from build123d import *

# Parameters (mm, degrees)
SKETCH1_W           = 200
SKETCH1_H           = 200
BOSS_EXTRUDE1_DEPTH = 340
CAVITY1_START       = -100
CAVITY1_DEPTH       = 200
CAVITY1_START_2     = 91.703376511
CAVITY1_2_DEPTH     = 8.296623489
CAVITY1_3_DEPTH     = 1.703376511


# Read off the part's stored shape, not the designer's step: Cavity1
with BuildPart() as part:
    # Sketch1 → Boss-Extrude1 (new body)
    with BuildSketch(Plane.XY):
        Rectangle(SKETCH1_W, SKETCH1_H)
    extrude(amount=BOSS_EXTRUDE1_DEPTH)

    # Cavity1 outline → Cavity1 (cut)
    with BuildSketch(Plane.YZ.offset(CAVITY1_START)):
        with BuildLine():
            ThreePointArc((100, 19.737266788), (79.748929914, 52.418363447), (64.730256288, 87.81044393))
            Line((64.730256288, 87.81044393), (43.715736742, 87.81044393))
            ThreePointArc((43.715736742, 87.81044393), (31.630726001, 167.81044393), (43.715736742, 247.81044393))
            Line((43.715736742, 247.81044393), (64.730256288, 247.81044393))
            ThreePointArc((64.730256288, 247.81044393), (79.748929914, 283.202524413), (100, 315.883621072))
            Line((100, 315.883621072), (100, 340))
            Line((100, 340), (-100, 340))
            Line((-100, 340), (-100, 0))
            Line((-100, 0), (100, 0))
            Line((100, 0), (100, 19.737266788))
        make_face()
    extrude(amount=CAVITY1_DEPTH, mode=Mode.SUBTRACT)

    # Cavity1 2 outline → Cavity1 2 (cut)
    with BuildSketch(Plane.YZ.offset(CAVITY1_START_2)):
        with BuildLine():
            Line((43.715736742, 87.81044393), (64.730256288, 87.81044393))
            ThreePointArc((64.730256288, 87.81044393), (79.748929914, 52.418363447), (100, 19.737266788))
            Line((100, 19.737266788), (100, 315.883621072))
            ThreePointArc((100, 315.883621072), (79.748929914, 283.202524413), (64.730256288, 247.81044393))
            Line((64.730256288, 247.81044393), (43.715736742, 247.81044393))
            ThreePointArc((43.715736742, 247.81044393), (31.630726001, 167.81044393), (43.715736742, 87.81044393))
        make_face()
    extrude(amount=CAVITY1_2_DEPTH, mode=Mode.SUBTRACT)

    # Cavity1 3 outline → Cavity1 3 (cut)
    with BuildSketch(Plane.YZ.offset(CAVITY1_START)):
        with BuildLine():
            Line((43.715736742, 87.81044393), (64.730256288, 87.81044393))
            ThreePointArc((64.730256288, 87.81044393), (79.748929914, 52.418363447), (100, 19.737266788))
            Line((100, 19.737266788), (100, 315.883621072))
            ThreePointArc((100, 315.883621072), (79.748929914, 283.202524413), (64.730256288, 247.81044393))
            Line((64.730256288, 247.81044393), (43.715736742, 247.81044393))
            ThreePointArc((43.715736742, 247.81044393), (31.630726001, 167.81044393), (43.715736742, 87.81044393))
        make_face()
    extrude(amount=CAVITY1_3_DEPTH, mode=Mode.SUBTRACT)


solid = part.part
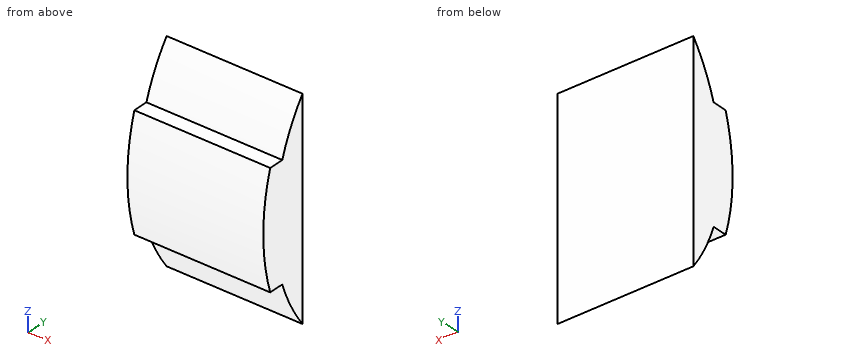
Could you check a few things on this model? Use its own coordinates, in mm. Give positions to 0.01 mm unless a question says otherwise; leave off trailing zeros. Order: outer loops, then holes, each group sorted by start corner. A loop starts at its lowest first (then second) coordinate and runs counter-clockwise, first axis right, second up.
1. Suppose I cut it at A-A (x = 33.5). Write out the boundary of the cut face in (y, z), plus the area to 3 significant figures.
Answers below:
outline: (43.72, 87.81) - (64.73, 87.81) arc R250.83 ccw to (100, 19.74) - (100, 315.88) arc R250.83 ccw to (64.73, 247.81) - (43.72, 247.81) arc R270.83 ccw to start
area: 13,000 mm2
2. I need wall thicknesses on L1, parallel to Z at x = 42.5, y = 58; L2, parallel to Y at x = -58.5, z = 171; L3, parallel to Y at x = 19.5, z = 278. Which ranges of each line are inside material? Lowest first, please.
Answers below:
L1: z = 87.81 to 247.81
L2: y = 31.65 to 100
L3: y = 77.13 to 100
3. Suppose I cut it at C-C (z = 281.5). Write out the boundary of the cut face in (x, y), plus the area to 3 significant figures.
Answers below:
outline: (-98.3, 78.88) - (91.7, 78.88) - (91.7, 100) - (-98.3, 100) - close
area: 4,010 mm2
4. Suppose I cut it at B-B (y = 58). Write out the boundary of the cut face in (x, z), plus the area to 3 significant figures.
Answers below:
outline: (-98.3, 87.81) - (91.7, 87.81) - (91.7, 247.81) - (-98.3, 247.81) - close
area: 30,400 mm2
5. For pin 1 (4 mm diameter, centred on x = 28.5, z = 278, fed in from -Y); pin 2 (12 mm diameter, centred on x = 51, y = 77.5, fed in from +Z); pin 3 (6.5 mm diameter, centred on x = -46, y = 59.5, fed in from +Z), each with a flat end and sliding along its axis, tell me the tip position at first contact or that it passes through.
Answers below:
pin 1: stops at y = 76.16
pin 2: stops at z = 290.17
pin 3: stops at z = 247.81
